Here's how the part is built. I have some questions about the finished solid (model axes, mm). Give positions to 0.01 mm unless a question says otherwise; leave off trailing zeros. Write each loop counter-clockwise with the first axis right and the second up, starting at its lowest first coordinate (ties: lowest second). Pieces come first, ordered by that corner, then holes. Notation, with made-up numbers: (20.25, 85.5) - (45.25, 85.5) arc R25 ccw to (45.25, 105.5) - close; hole circle Ø9 at (62, -38.5). An arc over 180 degrees is marked (long way). Write each question's results on one line, items separated by ' | '. Start each with the question number.
Item 1: Suppose I cut it at B-B on y = -31.75. List the corners of the cut face in (x, z) for me (3 decimals).
Item 2: We'd pull the mould along X, two halves only. Please class faces 1 (the flat face through (69.85, 4, 2)), 2 (the cylindrical face through (-1.21, -29.853, 1.553)), 3 (the flat face through (17, 15, 0)): +X half, -X half, draft (parallel to the pull), parting line (faces both ways), or undercut.
Item 3: Suppose I cut it at D-D on x = -63.5. List the corners of the cut face in (y, z) for me (3 decimals).
Item 4: Suppose I cut it at A-A on y = 0. Count the separate pieces of the cut face and the enclosed holes in it, then the cut area to 3 significant figures.
Item 5: Please list where these lines run through material, in increasing order: line 1 along X through (y, z) = (-31.75, 2.3); line 2 along Y through (x, z) = (0, 1.55) (3 decimals); line 3 along X through (y, z) = (30.5, 0.9).
Item 6: Will this pin go through, and if not, where does the flat tip stop? P1, Ø3.5, axis at x = -63.5, y = 31.75, coming from the +Z side.
```python
from build123d import *

# Parameters (mm, degrees)
BOSS_EXTRUDE1_DEPTH            = 3.175
M4_CLEARANCE_HOLE1_D           = 4.5
M4_CLEARANCE_HOLE1_CSINK_D     = 4.55
M4_CLEARANCE_HOLE1_CSINK_ANGLE = 90
M8_CLEARANCE_HOLE1_AT_2_COUNT  = 2
M8_CLEARANCE_HOLE1_AT_2_PITCH  = 84
SKETCH9_R                      = 21.275
CENTER_HOLE_DEPTH              = 85.39355735


with BuildPart() as part:
    # Sketch1 → Boss-Extrude1 (new body)
    with BuildSketch(Plane.XY):
        Polygon((-69.85, 38.1), (69.85, 47.256421755), (69.85, 38.1), (69.85, -38.1), (-69.85, -38.1), align=None)
    extrude(amount=BOSS_EXTRUDE1_DEPTH)

    # M4 Clearance Hole1 (through all)
    with Locations(Plane.XY.offset(3.175)):
        with Locations((-63.5, -31.75), (0, -31.75), (63.5, -31.75), (63.5, 31.75), (63.5, 0), (0, 31.75), (-63.5, 31.75), (-63.5, 0)):
            CounterSinkHole(M4_CLEARANCE_HOLE1_D / 2, M4_CLEARANCE_HOLE1_CSINK_D / 2, counter_sink_angle=M4_CLEARANCE_HOLE1_CSINK_ANGLE)

    # Sketch11 → M8 Clearance Hole1 (revolve, cut)
    with BuildSketch(Plane(origin=(-42, 0, 3.175), x_dir=(0, -1, 0), z_dir=(1, 0, 0))):
        Polygon((0, 0), (0, 3.175), (4.5, 3.175), (4.5, 0.025), (4.525, 0), align=None)
    m8_clearance_hole1 = revolve(axis=Axis((-42, 0, 9.525), (0, 0, -1)), mode=Mode.SUBTRACT)

    # M8 Clearance Hole1 at 2: M8 Clearance Hole1 ×2
    with Locations(*[(i * M8_CLEARANCE_HOLE1_AT_2_PITCH, 0, 0) for i in range(1, M8_CLEARANCE_HOLE1_AT_2_COUNT)]):
        add(m8_clearance_hole1, mode=Mode.SUBTRACT)

    # Sketch9 → Center Hole (cut, through all)
    with BuildSketch(Plane.XY.offset(3.175)):
        Circle(SKETCH9_R)
    extrude(amount=-CENTER_HOLE_DEPTH, mode=Mode.SUBTRACT)


solid = part.part
```
Checked values:
1) outline: (-69.85, 0) - (-65.75, 0) - (-65.75, 3.15) - (-65.775, 3.175) - (-69.85, 3.175) - close; (-61.25, 0) - (-2.25, 0) - (-2.25, 3.15) - (-2.275, 3.175) - (-61.225, 3.175) - (-61.25, 3.15) - close; (2.25, 0) - (61.25, 0) - (61.25, 3.15) - (61.225, 3.175) - (2.275, 3.175) - (2.25, 3.15) - close; (65.75, 0) - (69.85, 0) - (69.85, 3.175) - (65.775, 3.175) - (65.75, 3.15) - close
2) face 1: +X half | face 2: undercut | face 3: draft
3) outline: (-38.1, 0) - (-34, 0) - (-34, 3.15) - (-34.025, 3.175) - (-38.1, 3.175) - close; (-29.5, 0) - (-2.25, 0) - (-2.25, 3.15) - (-2.275, 3.175) - (-29.475, 3.175) - (-29.5, 3.15) - close; (2.25, 0) - (29.5, 0) - (29.5, 3.15) - (29.475, 3.175) - (2.275, 3.175) - (2.25, 3.15) - close; (34, 0) - (38.516, 0) - (38.516, 3.175) - (34.025, 3.175) - (34, 3.15) - close
4) separate pieces: 6 | enclosed holes: 0 | area: 223 mm^2
5) line 1: x = -69.85 to -65.75, -61.25 to -2.25, 2.25 to 61.25, 65.75 to 69.85 | line 2: y = -38.1 to -34, -29.5 to -21.275, 21.275 to 29.5, 34 to 42.678 | line 3: x = -69.85 to -65.37, -61.63 to -1.87, 1.87 to 61.63, 65.37 to 69.85
6) P1: passes through
